Work out the finished part from the listing and answer in its coordinate system (mm). A direction names the side the tool comes from. Coordinates: 2 decimals unless noted, no trailing zeros. Order: outer loops, then holes, each group sorted by start corner. A loop starts at its lowest first (then second) coordinate and runs counter-clockwise, first axis right, second up. Notation, with made-up numbers: M -25,61.25 L 20,61.25 A9 ccw 20,78.25 Z; hole C -9,13.25 d11. An arc over 180 degrees is marked long. Use a Markdown table: item, result.
from build123d import *

# Parameters (mm, degrees)
F2_DEPTH = 50
F4_R     = 2
F5_DEPTH = 2
F6_DEPTH = 4.8


with BuildPart() as f2:
    # F1 (on Front) → F2 (new body)
    with BuildSketch(Plane.XZ):
        Polygon((0, 19.8), (0, 0), (2, 0), (2, 15), (30, 15), (30, 19.8), align=None)
    extrude(amount=-F2_DEPTH)

    # F4 (on face) → F5 (cut, through all)
    with BuildSketch(Plane(origin=(0, 0, 0), x_dir=(0, -1, 0), z_dir=(-1, 0, 0))):
        with Locations((-25, 10)):
            Circle(F4_R)
    extrude(amount=-F5_DEPTH, mode=Mode.SUBTRACT)

    # F3 (on face) → F6 (cut, through all)
    with BuildSketch(Plane.XY.offset(19.8)):
        with BuildLine():
            ThreePointArc((19, 21.8), (18.9292893219, 21.6292893219), (19.1, 21.7))
            Line((19.1, 21.7), (19, 21.7))
            Line((19, 21.7), (19, 21.8))
        make_face()
        with BuildLine():
            ThreePointArc((19, 21.8), (19.0707106781, 21.7707106781), (19.1, 21.7))
            Line((19.1, 21.7), (23.9, 21.7))
            ThreePointArc((23.9, 21.7), (23.9292893219, 21.7707106781), (24, 21.8))
            Line((24, 21.8), (24, 28.2))
            ThreePointArc((24, 28.2), (23.9292893219, 28.2292893219), (23.9, 28.3))
            Line((23.9, 28.3), (19.1, 28.3))
            ThreePointArc((19.1, 28.3), (19.0707106781, 28.2292893219), (19, 28.2))
            Line((19, 28.2), (19, 21.8))
        make_face()
        with BuildLine():
            Line((19, 21.7), (19.1, 21.7))
            ThreePointArc((19.1, 21.7), (19.0707106781, 21.7707106781), (19, 21.8))
            Line((19, 21.8), (19, 21.7))
        make_face()
        with BuildLine():
            ThreePointArc((24, 21.8), (23.9292893219, 21.7707106781), (23.9, 21.7))
            Line((23.9, 21.7), (24, 21.7))
            Line((24, 21.7), (24, 21.8))
        make_face()
        with BuildLine():
            Line((24, 21.7), (23.9, 21.7))
            ThreePointArc((23.9, 21.7), (24, 21.6), (24.1, 21.7))
            ThreePointArc((24.1, 21.7), (24.0707106781, 21.7707106781), (24, 21.8))
            Line((24, 21.8), (24, 21.7))
        make_face()
        with BuildLine():
            ThreePointArc((19.1, 28.3), (18.9292893219, 28.3707106781), (19, 28.2))
            Line((19, 28.2), (19, 28.3))
            Line((19, 28.3), (19.1, 28.3))
        make_face()
        with BuildLine():
            Line((19, 28.3), (19, 28.2))
            ThreePointArc((19, 28.2), (19.0707106781, 28.2292893219), (19.1, 28.3))
            Line((19.1, 28.3), (19, 28.3))
        make_face()
        with BuildLine():
            ThreePointArc((23.9, 28.3), (23.9292893219, 28.2292893219), (24, 28.2))
            Line((24, 28.2), (24, 28.3))
            Line((24, 28.3), (23.9, 28.3))
        make_face()
        with BuildLine():
            Line((24, 28.3), (24, 28.2))
            ThreePointArc((24, 28.2), (24.0707106781, 28.2292893219), (24.1, 28.3))
            ThreePointArc((24.1, 28.3), (24, 28.4), (23.9, 28.3))
            Line((23.9, 28.3), (24, 28.3))
        make_face()
        with BuildLine():
            ThreePointArc((19, 37.8), (18.9292893219, 37.6292893219), (19.1, 37.7))
            Line((19.1, 37.7), (19, 37.7))
            Line((19, 37.7), (19, 37.8))
        make_face()
        with BuildLine():
            ThreePointArc((19, 37.8), (19.0707106781, 37.7707106781), (19.1, 37.7))
            Line((19.1, 37.7), (23.9, 37.7))
            ThreePointArc((23.9, 37.7), (23.9292893219, 37.7707106781), (24, 37.8))
            Line((24, 37.8), (24, 44.2))
            ThreePointArc((24, 44.2), (23.9292893219, 44.2292893219), (23.9, 44.3))
            Line((23.9, 44.3), (19.1, 44.3))
            ThreePointArc((19.1, 44.3), (19.0707106781, 44.2292893219), (19, 44.2))
            Line((19, 44.2), (19, 37.8))
        make_face()
        with BuildLine():
            Line((19, 37.7), (19.1, 37.7))
            ThreePointArc((19.1, 37.7), (19.0707106781, 37.7707106781), (19, 37.8))
            Line((19, 37.8), (19, 37.7))
        make_face()
        with BuildLine():
            ThreePointArc((24, 37.8), (23.9292893219, 37.7707106781), (23.9, 37.7))
            Line((23.9, 37.7), (24, 37.7))
            Line((24, 37.7), (24, 37.8))
        make_face()
        with BuildLine():
            Line((24, 37.7), (23.9, 37.7))
            ThreePointArc((23.9, 37.7), (24, 37.6), (24.1, 37.7))
            ThreePointArc((24.1, 37.7), (24.0707106781, 37.7707106781), (24, 37.8))
            Line((24, 37.8), (24, 37.7))
        make_face()
        with BuildLine():
            ThreePointArc((19.1, 44.3), (18.9292893219, 44.3707106781), (19, 44.2))
            Line((19, 44.2), (19, 44.3))
            Line((19, 44.3), (19.1, 44.3))
        make_face()
        with BuildLine():
            Line((19, 44.3), (19, 44.2))
            ThreePointArc((19, 44.2), (19.0707106781, 44.2292893219), (19.1, 44.3))
            Line((19.1, 44.3), (19, 44.3))
        make_face()
        with BuildLine():
            Line((24, 44.3), (24, 44.2))
            ThreePointArc((24, 44.2), (24.0707106781, 44.2292893219), (24.1, 44.3))
            ThreePointArc((24.1, 44.3), (24, 44.4), (23.9, 44.3))
            Line((23.9, 44.3), (24, 44.3))
        make_face()
        with BuildLine():
            ThreePointArc((23.9, 44.3), (23.9292893219, 44.2292893219), (24, 44.2))
            Line((24, 44.2), (24, 44.3))
            Line((24, 44.3), (23.9, 44.3))
        make_face()
        with BuildLine():
            ThreePointArc((19, 12.2), (19.0707106781, 12.2292893219), (19.1, 12.3))
            Line((19.1, 12.3), (19, 12.3))
            Line((19, 12.3), (19, 12.2))
        make_face()
        with BuildLine():
            Line((19, 12.3), (19.1, 12.3))
            ThreePointArc((19.1, 12.3), (18.9292893219, 12.3707106781), (19, 12.2))
            Line((19, 12.2), (19, 12.3))
        make_face()
        with BuildLine():
            Line((23.9, 12.3), (19.1, 12.3))
            ThreePointArc((19.1, 12.3), (19.0707106781, 12.2292893219), (19, 12.2))
            Line((19, 12.2), (19, 5.8))
            ThreePointArc((19, 5.8), (19.0707106781, 5.7707106781), (19.1, 5.7))
            Line((19.1, 5.7), (23.9, 5.7))
            ThreePointArc((23.9, 5.7), (23.9292893219, 5.7707106781), (24, 5.8))
            Line((24, 5.8), (24, 12.2))
            ThreePointArc((24, 12.2), (23.9292893219, 12.2292893219), (23.9, 12.3))
        make_face()
        with BuildLine():
            ThreePointArc((24.1, 12.3), (24, 12.4), (23.9, 12.3))
            Line((23.9, 12.3), (24, 12.3))
            Line((24, 12.3), (24, 12.2))
            ThreePointArc((24, 12.2), (24.0707106781, 12.2292893219), (24.1, 12.3))
        make_face()
        with BuildLine():
            Line((24, 12.3), (23.9, 12.3))
            ThreePointArc((23.9, 12.3), (23.9292893219, 12.2292893219), (24, 12.2))
            Line((24, 12.2), (24, 12.3))
        make_face()
        with BuildLine():
            ThreePointArc((19.1, 5.7), (19.0707106781, 5.7707106781), (19, 5.8))
            Line((19, 5.8), (19, 5.7))
            Line((19, 5.7), (19.1, 5.7))
        make_face()
        with BuildLine():
            Line((19, 5.7), (19, 5.8))
            ThreePointArc((19, 5.8), (18.9292893219, 5.6292893219), (19.1, 5.7))
            Line((19.1, 5.7), (19, 5.7))
        make_face()
        with BuildLine():
            Line((24, 5.7), (24, 5.8))
            ThreePointArc((24, 5.8), (23.9292893219, 5.7707106781), (23.9, 5.7))
            Line((23.9, 5.7), (24, 5.7))
        make_face()
        with BuildLine():
            ThreePointArc((24.1, 5.7), (24.0707106781, 5.7707106781), (24, 5.8))
            Line((24, 5.8), (24, 5.7))
            Line((24, 5.7), (23.9, 5.7))
            ThreePointArc((23.9, 5.7), (24, 5.6), (24.1, 5.7))
        make_face()
    extrude(amount=-F6_DEPTH, mode=Mode.SUBTRACT)


solid = f2.part
(1) Determine the mould class of faces 4 (the flat face through (1, 25, 0)), 5 (the flat face through (0, 24.6, 12.2)), 6 (the flat face through (22, 44.3, 17)) for opening direction X: pulls with the +X half, pulls with the -X half, needs draft (parallel to the pull), parting line crosses it, or undercut.
Conclusion:
| item | result |
|---|---|
| face 4 | needs draft |
| face 5 | pulls with the -X half |
| face 6 | undercut |
(2) Straight lines are drawn through the part: L1, parallel to Y at x = 19.5, z = 18.25; L2, parallel to Z at x = 1.35, y = 25; L3, parallel to Z at x = 28.5, y = 30.5. For each, find the intervals that lie inside material, in ascending order.
Conclusion:
| item | result |
|---|---|
| L1 | 0 to 5.7, 12.3 to 21.7, 28.3 to 37.7, 44.3 to 50 |
| L2 | 0 to 8, 12 to 19.8 |
| L3 | 15 to 19.8 |
(3) A cutting plane is placed at A-A (y = 9.5). Determine the outline of the cut face in (x, z), then the cut area to 3 significant figures.
Conclusion:
| item | result |
|---|---|
| outline | M 0,0 L 2,0 L 2,15 L 19,15 L 19,19.8 L 0,19.8 Z; M 24,15 L 30,15 L 30,19.8 L 24,19.8 Z |
| area | 150 mm2 |
(4) A cutting plane is placed at B-B (z = 10). Determine the outline of the cut face in (x, y), then the cut area to 3 significant figures.
Conclusion:
| item | result |
|---|---|
| outline | M 0,0 L 2,0 L 2,23 L 0,23 Z; M 0,27 L 2,27 L 2,50 L 0,50 Z |
| area | 92.0 mm2 |
(5) A cutting plane is placed at C-C (y = 25). Determine the outline of the cut face in (x, z), then the cut area to 3 significant figures.
Conclusion:
| item | result |
|---|---|
| outline | M 0,0 L 2,0 L 2,8 L 0,8 Z; M 0,12 L 2,12 L 2,15 L 19,15 L 19,19.8 L 0,19.8 Z; M 24,15 L 30,15 L 30,19.8 L 24,19.8 Z |
| area | 142 mm2 |
(6) Which of the six approach directions +Z, -Z, +X, -X, +Y, -Y give full straight-line access (tool end or side, diameter ignored) to faces 1 (the flat face through (2, 25, 7)), 2 (the flat face through (12, 0, 17)), 3 (the flat face through (21, 5.7, 17))?
Conclusion:
| item | result |
|---|---|
| face 1 | -Z, +X, +Y, -Y |
| face 2 | +Z, -Z, +X, -X, -Y |
| face 3 | +Z, -Z |
(7) Given P1, Ø10, axis at y = 39, z = 17.5, coming from the -X side; P2, Ø2.5, axis at y = 25, z = 10, coming from the -X side (3 decimals); P3, Ø8, axis at y = 18.5, z = 9, coming from the +X side, each flat-ended and moving along its own axis, determine where each tip first touches the part or whether it passes through.
Conclusion:
| item | result |
|---|---|
| P1 | x = 0 |
| P2 | through |
| P3 | x = 2 |
(8) A cutting plane is placed at D-D (x = 12.75). Determine the outline of the cut face in (y, z), then the cut area to 3 significant figures.
Conclusion:
| item | result |
|---|---|
| outline | M 0,15 L 50,15 L 50,19.8 L 0,19.8 Z |
| area | 240 mm2 |
